Input: dimensioned drawing with shaded views. Units: mm. Origin: part minimum x, y, z. A direction names the side the tool comes from. Round coordinates to 2 decimals unless told otherwise and drop trailing zeros. Order: outer loops, then holes, each group sorted by start corner. A loop starts at its lowest first (then second) coordinate and runs counter-clockwise, first axis right, second up. Notation, with made-up numbers: M 45,67.5 L 70,67.5 A13 cw 70,78.5 Z; hole C 26.5,-14 d6. An arc over 180 degrees is marked long. Put each result on its own line as item: value. Start each with the question number.
1) Section B-B, the plane y = 2. Return loops of the section in (x, z), then the cut area to 3 significant figures.
2) Access query for the marked faces 1, 2 and 3. Directions: +Z, -Z, +X, -X, +Y, -Y. A direction counts if a zero-diameter tool reaches every point of the face in a straight line with its end or side. Return the directions, or none.
3) Material intervals for probe 1 along Z at (x, y) = (3.15, 2.4); probe 2 along Z at (x, y) = (2.9, 3.25); probe 3 along Y at (x, z) = (3.8, 11), sorted ascending. Write a range as [from, to].
4) Section C-C, the plane x = 0.3. Return loops of the section in (y, z).
5) Section A-A, the plane x = 2. Return loops of the section in (y, z).
6) Section D-D, the plane y = 0.8. Return loops of the section in (x, z).
7) Draft query along Z for the marked faces 4, 5, 6 and 7. Return one class per face: pulls with the +Z half, pulls with the -Z half, needs draft (parallel to the pull), parting line crosses it, or undercut.
8) First-contact query: P1, Ø1, axis at y = 0.5, z = 10.5, coming from the +X side; P2, Ø2, axis at y = 0.5, z = 4.5, coming from the +X side; P3, Ø1.5, axis at y = 1, z = 4.5, coming from the +X side. Flat tips, straight axial feed; report the tip coordinate or a pass-through.
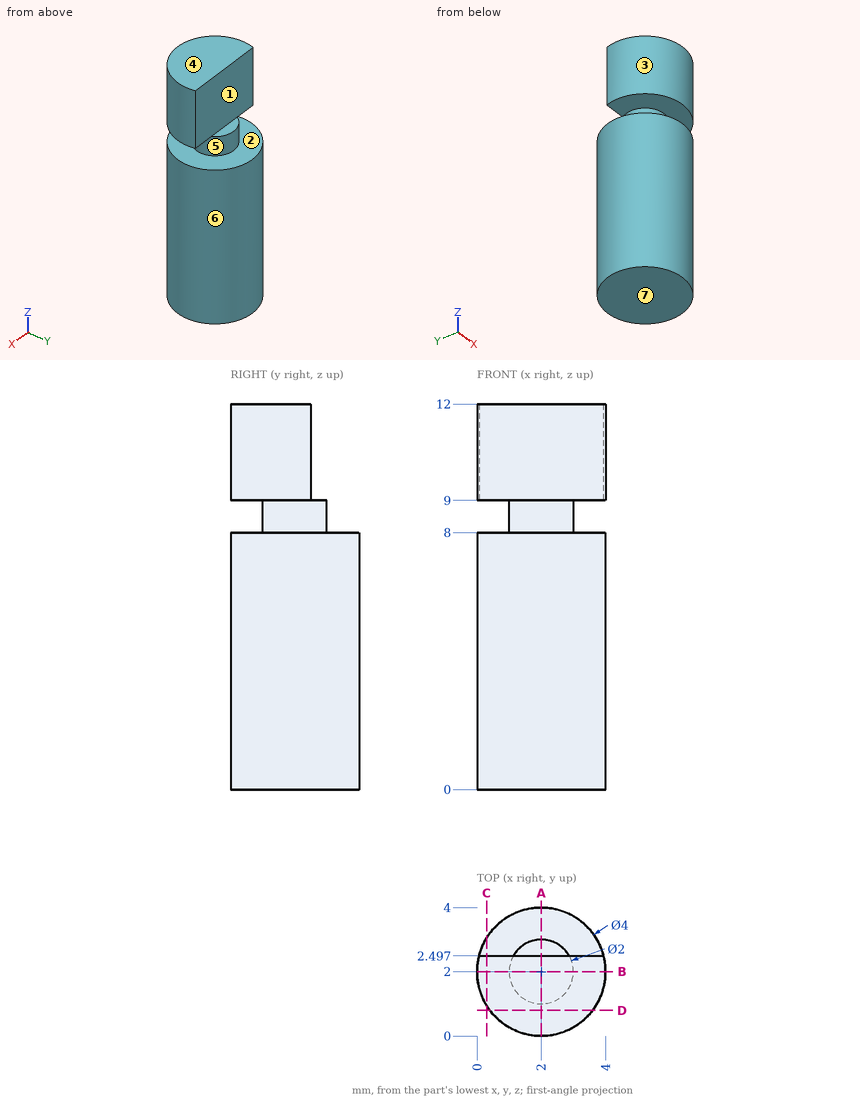
Result sheet:
1. outline: M 0,0 L 4,0 L 4,8 L 3,8 L 3,9 L 4,9 L 4,12 L 0,12 L 0,9 L 1,9 L 1,8 L 0,8 Z
1. area: 46.0 mm2
2. face 1: +Z, +X, -X, +Y
2. face 2: none
2. face 3: +Z, -Z
3. probe 1: z = [0, 8], [9, 12]
3. probe 2: z = [0, 8]
3. probe 3: y = [1.13, 2.5]
4. outline: M 0.95,0 L 3.05,0 L 3.05,8 L 0.95,8 Z; M 0.95,9 L 2.5,9 L 2.5,12 L 0.95,12 Z
5. outline: M 0,0 L 4,0 L 4,8 L 3,8 L 3,9 L 2.5,9 L 2.5,12 L 0,12 L 0,9 L 1,9 L 1,8 L 0,8 Z
6. outline: M 0.4,0 L 3.6,0 L 3.6,8 L 0.4,8 Z; M 0.4,9 L 3.6,9 L 3.6,12 L 0.4,12 Z
7. face 4: pulls with the +Z half
7. face 5: undercut
7. face 6: needs draft
7. face 7: pulls with the -Z half
8. P1: stops at x = 3.73
8. P2: stops at x = 3.94
8. P3: stops at x = 3.98
